For this review, take the finished solid that the model builds, in its own axes (mm). A direction names the side the tool comes from. Give positions to 0.01 mm unless a question says otherwise; leave off trailing zeros. Order: outer loops, then holes, each group sorted by start corner. A loop starts at its lowest first (then second) coordinate and runs counter-clockwise, first axis right, second up.
Item 1: Consider section B-B (y = 62). Give the boundary of the cut face in (x, z), plus the area to 3 significant figures.
Item 2: Machinability: for faces 1 (the flat face through (-48.051, -26.773, 1.972)), 2 (the flat face through (-169.76, -50.67, 1.97)), 3 (the flat face through (128.758, -121.681, 1.972)), which of the approach directions +Z, -Z, +X, -X, +Y, -Y give a long, thin tool a straight path to every point of the face, cutting with its end or side? Answer none if there is none.
Item 3: The part is to be moulded in two halves that separate along X. For faces 4 (the cylindrical face through (-172.034, 102.002, 1.972)), 5 (the cylindrical face through (174.353, 97.985, 1.972)), 6 (the cylindrical face through (13.887, 10.648, 1.972)), say which applies: released by +X, released by -X, zero draft, split by the parting line, or undercut.
Item 4: Consider section C-C (x = -173). Give the boundary of the cut face in (y, z), plus the area to 3 significant figures.
Item 5: Consider section D-D (z = 2.45). Give the number of separate pieces and of enclosed holes in the cut face, plus the area to 3 significant figures.
Item 6: Consider section A-A (x = 0). Give the boundary of the cut face in (y, z).
Item 7: For P1, Ø2, axis at x = 2.5, z = 2, coming from the +Y side; P2, Ø4, axis at x = -98.28, y = -122.23, coming from the -Z side; P3, Ø4, axis at x = -132.51, y = 89.49, coming from the -Z side; P4, Ø1.5, axis at y = -143, z = 0.5, coming from the -X side, all flat-tipped, find the tip position at first contact; note any pin that passes through.
Item 8: For probe 1 along Y at (x, z) = (71, 3); probe 2 along X at (y, z) = (18.5, 1.3); probe 3 along X at (y, z) = (-146, 3.65), list the stretches that pass through material, from the lowest coordinate up.
```python
from build123d import *

# Parameters (mm, degrees)
SKETCH1_R           = 200
BOSS_EXTRUDE2_DEPTH = 4
CUT_EXTRUDE3_DEPTH  = 4
SKETCH4_R           = 17.500000000000004
CUT_EXTRUDE4_DEPTH  = 4
SKETCH5_R           = 2
CUT_EXTRUDE5_DEPTH  = 4
SKETCH6_R           = 1.4999999999999973
SKETCH6_R_2         = 1.5000000000000042
CUT_EXTRUDE6_DEPTH  = 4
CIRPATTERN2_COUNT   = 3
CIRPATTERN3_COUNT   = 3
CUT_EXTRUDE7_DEPTH  = 4
CIRPATTERN4_COUNT   = 3
SKETCH9_R           = 3.500000000000001
SKETCH9_R_2         = 3.5000000000000075
CUT_EXTRUDE8_DEPTH  = 4
CIRPATTERN5_COUNT   = 3
CIRPATTERN6_COUNT   = 3
FILLET1_R           = 2
FILLET2_R           = 2


with BuildPart() as part:
    # Sketch1 → Boss-Extrude2 (new body)
    with BuildSketch(Plane.XY):
        Circle(SKETCH1_R)
    extrude(amount=BOSS_EXTRUDE2_DEPTH)

    # Sketch3 → Cut-Extrude3 (cut)
    with BuildSketch(Plane.XY):
        with BuildLine():
            Line((-41.00000000000001, 195.75239462136855), (-41, 150.00000000000003))
            Line((-41, 150.00000000000003), (41, 150.00000000000003))
            Line((41, 150.00000000000003), (41.00000000000001, 195.75239462136855))
            ThreePointArc((41.00000000000001, 195.75239462136855), (1.225e-14, 200), (-41.00000000000001, 195.75239462136855))
        make_face()
    cut_extrude3 = extrude(amount=CUT_EXTRUDE3_DEPTH, mode=Mode.SUBTRACT)

    # Sketch4 → Cut-Extrude4 (cut)
    with BuildSketch(Plane.XY):
        with Locations(Location((0, 0, 0), (0, 0, 180))):
            Circle(SKETCH4_R)
    extrude(amount=CUT_EXTRUDE4_DEPTH, mode=Mode.SUBTRACT)

    # Sketch5 → Cut-Extrude5 (cut)
    with BuildSketch(Plane.XY):
        with Locations(Location((-20, 136, 0), (0, 0, 180))):
            Circle(SKETCH5_R)
        with Locations(Location((-20, 95, 0), (0, 0, 180))):
            Circle(SKETCH5_R)
        with Locations(Location((20, 136, 0), (0, 0, 180))):
            Circle(SKETCH5_R)
        with Locations(Location((20, 95, 0), (0, 0, 180))):
            Circle(SKETCH5_R)
    cut_extrude5 = extrude(amount=CUT_EXTRUDE5_DEPTH, mode=Mode.SUBTRACT)

    # Sketch6 → Cut-Extrude6 (cut)
    with BuildSketch(Plane.XY):
        with Locations((-143.75605190361796, 70.00721420742511)):
            Circle(SKETCH6_R)
        with Locations((-132.50605190361796, 89.49278579257494)):
            Circle(SKETCH6_R)
        with Locations((-35.94421938165304, 33.742785792574935)):
            Circle(SKETCH6_R_2)
        with Locations((-47.19421938165304, 14.257214207425067)):
            Circle(SKETCH6_R_2)
    cut_extrude6 = extrude(amount=CUT_EXTRUDE6_DEPTH, mode=Mode.SUBTRACT)

    # CirPattern2: Cut-Extrude6 ×3 about axis
    cirpattern2_axis = Axis((9.38e-15, 1.23e-15, 0), (0, 0, 1))
    for i in range(1, CIRPATTERN2_COUNT):
        add(cut_extrude6.rotate(cirpattern2_axis, i * 360 / CIRPATTERN2_COUNT), mode=Mode.SUBTRACT)

    # CirPattern3: Cut-Extrude5 ×3 about axis
    cirpattern3_axis = Axis((6.55e-15, -6.68e-15, 0), (0, 0, 1))
    for i in range(1, CIRPATTERN3_COUNT):
        add(cut_extrude5.rotate(cirpattern3_axis, i * 360 / CIRPATTERN3_COUNT), mode=Mode.SUBTRACT)

    # Sketch8 → Cut-Extrude7 (cut)
    with BuildSketch(Plane.XY):
        with BuildLine():
            Line((-60, 69), (60, 69.00000000000003))
            ThreePointArc((60, 69.00000000000003), (66.99999999999997, 62), (60, 55.00000000000002))
            Line((60, 55.00000000000002), (-60, 55))
            ThreePointArc((-60, 55), (-67, 62), (-60, 69))
        make_face()
    cut_extrude7 = extrude(amount=CUT_EXTRUDE7_DEPTH, mode=Mode.SUBTRACT)

    # CirPattern4: Cut-Extrude7 ×3 about axis
    cirpattern4_axis = Axis((2.08e-15, -4.82e-15, 0), (0, 0, 1))
    for i in range(1, CIRPATTERN4_COUNT):
        add(cut_extrude7.rotate(cirpattern4_axis, i * 360 / CIRPATTERN4_COUNT), mode=Mode.SUBTRACT)

    # Sketch9 → Cut-Extrude8 (cut)
    with BuildSketch(Plane.XY.offset(4)):
        with Locations((-56.71539030917355, 146.233937586588)):
            Circle(SKETCH9_R)
        with Locations((-98.28460969082658, 122.23393758658793)):
            Circle(SKETCH9_R_2)
        Polygon((-91.16025403784447, 137.89419162443235), (-81.16025403784445, 120.57368354874356), (-63.83974596215569, 130.57368354874362), (-73.8397459621557, 147.89419162443235), align=None)
        with BuildLine():
            Line((-64.46891108675452, 118.66342951089922), (-60.46891108675456, 111.73522628062365))
            ThreePointArc((-60.46891108675456, 111.73522628062365), (-61.75000000000001, 106.9541373673781), (-66.53108891324563, 108.23522628062368))
            Line((-66.53108891324563, 108.23522628062368), (-70.53108891324557, 115.1634295108992))
            ThreePointArc((-70.53108891324557, 115.1634295108992), (-69.25000000000003, 119.94451842414472), (-64.46891108675452, 118.66342951089922))
        make_face()
        with BuildLine():
            Line((-84.46891108675456, 153.30444566227675), (-88.46891108675459, 160.23264889255222))
            ThreePointArc((-88.46891108675459, 160.23264889255222), (-93.25000000000009, 161.5137378057978), (-94.53108891324563, 156.73264889255222))
            Line((-94.53108891324563, 156.73264889255222), (-90.53108891324563, 149.80444566227675))
            ThreePointArc((-90.53108891324563, 149.80444566227675), (-85.7500000000001, 148.52335674903122), (-84.46891108675456, 153.30444566227675))
        make_face()
    cut_extrude8 = extrude(amount=-CUT_EXTRUDE8_DEPTH, mode=Mode.SUBTRACT)

    # CirPattern5: Cut-Extrude8 ×3 about axis
    cirpattern5_axis = Axis((6.83e-15, -3.41e-15, 0), (0, 0, 1))
    for i in range(1, CIRPATTERN5_COUNT):
        add(cut_extrude8.rotate(cirpattern5_axis, i * 360 / CIRPATTERN5_COUNT), mode=Mode.SUBTRACT)

    # CirPattern6: Cut-Extrude3 ×3 about axis
    cirpattern6_axis = Axis((-9.9e-16, -1.19e-14, 0), (0, 0, 1))
    for i in range(1, CIRPATTERN6_COUNT):
        add(cut_extrude3.rotate(cirpattern6_axis, i * 360 / CIRPATTERN6_COUNT), mode=Mode.SUBTRACT)

    # Fillet1
    fillet1_edges = [part.edges().sort_by_distance(p)[0] for p in [
        (41.00000000000001, 195.75239462136855, 2),
        (-41.00000000000001, 195.75239462136855, 2),
        (-41, 150.00000000000003, 2),
        (41, 150.00000000000003, 2),
        (149.0265465937414, -133.38323886584638, 2),
        (190.02654659374144, -62.36915575552241, 2),
        (150.4038105676658, -39.49295844483813, 2),
        (109.40381056766577, -110.50704155516208, 2),
        (-190.0265465937415, -62.36915575552226, 2),
        (-149.0265465937415, -133.38323886584627, 2),
        (-109.40381056766586, -110.50704155516199, 2),
        (-150.40381056766583, -39.49295844483801, 2),
    ]]
    fillet(fillet1_edges, radius=FILLET1_R)

    # Fillet2
    fillet2_edges = [part.edges().sort_by_distance(p)[0] for p in [
        (-91.16025403784447, 137.89419162443235, 2),
        (-73.8397459621557, 147.89419162443235, 2),
        (-63.83974596215569, 130.57368354874362, 2),
        (-81.16025403784445, 120.57368354874356, 2),
        (-73.83974596215556, -147.8941916244324, 2),
        (-91.16025403784433, -137.8941916244324, 2),
        (-81.16025403784437, -120.57368354874366, 2),
        (-63.83974596215556, -130.57368354874362, 2),
        (165.00000000000003, 10, 2),
        (165, -10, 2),
        (145.00000000000006, -10.000000000000014, 2),
        (145, 10, 2),
    ]]
    fillet(fillet2_edges, radius=FILLET2_R)


solid = part.part
```
Resolved:
1. outline: (-190.15, 0) - (-67, 0) - (-67, 4) - (-190.15, 4) - close; (67, 0) - (190.15, 0) - (190.15, 4) - (67, 4) - close
1. area: 985 mm2
2. face 1: +Z, -Z
2. face 2: +Z, -Z, -Y
2. face 3: +Z, -Z, +X
3. face 4: released by -X
3. face 5: released by +X
3. face 6: undercut
4. outline: (-52.54, 0) - (100.35, 0) - (100.35, 4) - (-52.54, 4) - close
4. area: 612 mm2
5. separate pieces: 1
5. enclosed holes: 43
5. area: 105,000 mm2
6. outline: (-200, 0) - (-17.5, 0) - (-17.5, 4) - (-200, 4) - close; (17.5, 0) - (55, 0) - (55, 4) - (17.5, 4) - close; (69, 0) - (150, 0) - (150, 4) - (69, 4) - close
7. P1: stops at y = 150
7. P2: passes through
7. P3: stops at z = 0
7. P4: stops at x = -140.59
8. probe 1: y = -186.97 to -66.36, -63.28 to -15.02, 12.98 to 186.97
8. probe 2: x = -199.14 to -90.25, -74.19 to 74.19, 90.25 to 199.14
8. probe 3: x = -136.69 to -77.12, -72.75 to -60.21, -53.22 to 136.69
